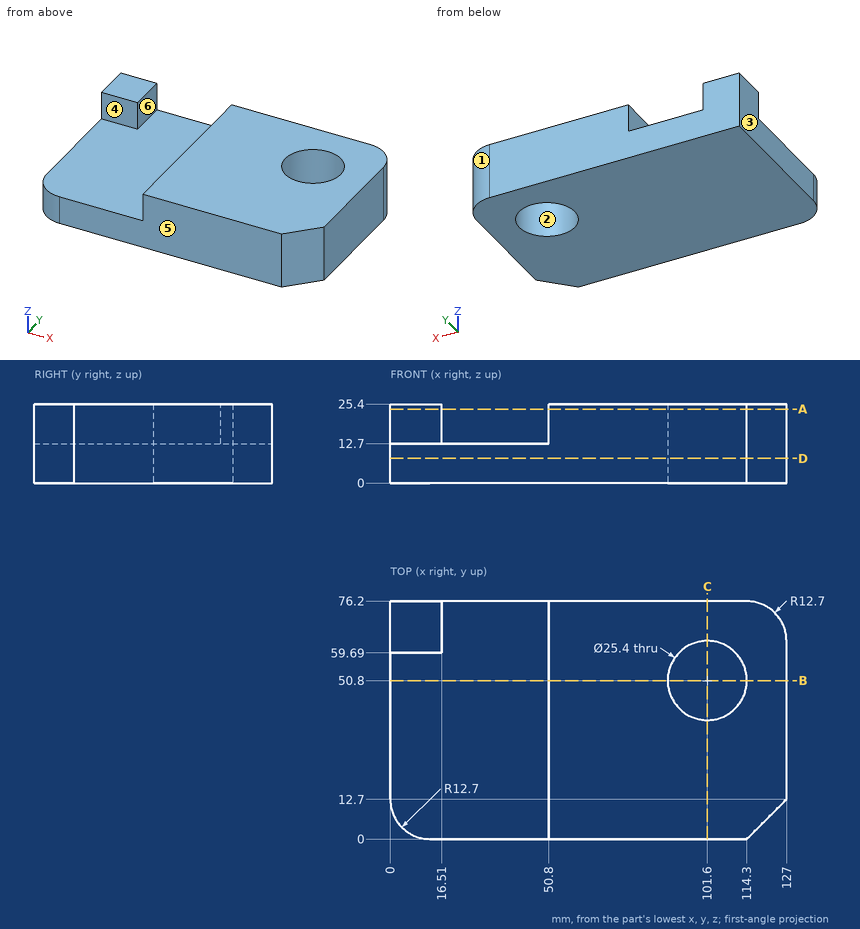
The figure shows three views and two pictorial views of one solid part (mm, origin at its lowest corner). Answer the questions. A direction names the side the tool comes from. Coordinates: 2 decimals unless noted, no trailing zeros. Write each loop counter-clockwise with the first axis right and the second up, starting at its lowest first coordinate (ties: lowest second). Pieces come first, ordered by that corner, then holes.
1. Flat-ended cylindrical pins translate along their axes: pin 1 (15 mm diameter, centred on x = 37, y = 22, fed in from +Z); pin 2 (10 mm diameter, centred on y = 54, z = 19.5, fed in from -X); pin 3 (6.5 mm diameter, centred on x = 10, z = 22, fed in from -Y). Find the tip coordinate at first contact, or state that the pin passes through.
Results list:
pin 1: stops at z = 12.7
pin 2: stops at x = 50.8
pin 3: stops at y = 59.69
2. For the marked faces 5 and 6, determine the directions among +Z, -Z, +X, -X, +Y, -Y from which every point of the face is accessible in a straight line to the end or side of a thin tool.
Results list:
face 5: +Z, -Z, +X, -X, -Y
face 6: +Z, +Y, -Y
3. Consider line 1 along X through (y, z) = (60, 18.5) (3 decimals); line 2 along Y through (x, z) = (101.6, 13.25); line 3 along Z through (x, y) = (6, 17). Determine where each line is inside the solid, lowest interval first.
Results list:
line 1: x = 0 to 16.51, 50.8 to 92.845, 110.355 to 127
line 2: y = 0 to 38.1, 63.5 to 76.2
line 3: z = 0 to 12.7
4. The part is cut by section A-A, the plane z = 23.75. Write down the section's boundary in (x, y), and give its area (3 significant figures).
Results list:
outline: (0, 59.69) - (16.51, 59.69) - (16.51, 76.2) - (0, 76.2) - close; (50.8, 0) - (114.3, 0) - (127, 12.7) - (127, 63.5) arc R12.7 ccw to (114.3, 76.2) - (50.8, 76.2) - close; hole circle Ø25.4 at (101.6, 50.8)
area: 5,460 mm2
5. The part is cut by section D-D, the plane z = 8. Write down the section's boundary in (x, y), and give its area (3 significant figures).
Results list:
outline: (0, 12.7) arc R12.7 ccw to (12.7, 0) - (114.3, 0) - (127, 12.7) - (127, 63.5) arc R12.7 ccw to (114.3, 76.2) - (0, 76.2) - close; hole circle Ø25.4 at (101.6, 50.8)
area: 9,020 mm2
6. For a pull along X with two mould halves and no side action, classify the marked faces 1, 2, 3 and 4 as +X half, -X half, draft (parallel to the pull), parting line (faces both ways), or undercut.
Results list:
face 1: +X half
face 2: undercut
face 3: -X half
face 4: draft
7. The part is cut by section C-C, the plane x = 101.6. Write down the section's boundary in (y, z).
Results list:
outline: (0, 0) - (38.1, 0) - (38.1, 25.4) - (0, 25.4) - close; (63.5, 0) - (76.2, 0) - (76.2, 25.4) - (63.5, 25.4) - close
8. The part is cut by section B-B, the plane y = 50.8. Write down the section's boundary in (x, z).
Results list:
outline: (0, 0) - (88.9, 0) - (88.9, 25.4) - (50.8, 25.4) - (50.8, 12.7) - (0, 12.7) - close; (114.3, 0) - (127, 0) - (127, 25.4) - (114.3, 25.4) - close
